Read the model definition and answer for the solid it produces. Units are mm, in the model's axes. Coordinates: 2 decimals unless noted, no trailing zeros. Write each loop counter-clockwise with the first axis right and the second up, starting at its lowest first coordinate (ties: lowest second). Pieces come first, ordered by that corner, then holes. Notation, with made-up numbers: M 83,74 L 114,74 A12 ccw 114,97 Z; hole C 69.5,-6 d8. An arc over 180 degrees is marked long. Write item = value, one per line.
from build123d import *

# Parameters (mm, degrees)
SKETCH1_R           = 4
BOSS_EXTRUDE1_DEPTH = 7
SKETCH2_R           = 3.375
CUT_EXTRUDE1_DEPTH  = 10
BOSS_EXTRUDE2_START = -0.25
SKETCH16_R          = 4.25
SKETCH16_R_2        = 4
BOSS_EXTRUDE2_DEPTH = 0.25


with BuildPart() as part:
    # Sketch1 → Boss-Extrude1 (new body)
    with BuildSketch(Plane(origin=(0, 0, 0), x_dir=(1, 0, 0), z_dir=(0, 1, 0))):
        with Locations(Location((0, 0, 0), (0, 0, 270))):
            Circle(SKETCH1_R)
    extrude(amount=BOSS_EXTRUDE1_DEPTH)

    # Sketch2 → Cut-Extrude1 (cut)
    with BuildSketch(Plane(origin=(0, 7, 0), x_dir=(1, 0, 0), z_dir=(0, 1, 0))):
        with Locations(Location((0, 0, 0), (0, 0, 270))):
            Circle(SKETCH2_R)
    extrude(amount=-CUT_EXTRUDE1_DEPTH, mode=Mode.SUBTRACT)

    # Sketch16 → Boss-Extrude2 (add)
    with BuildSketch(Plane(origin=(0, 7, 0), x_dir=(1, 0, 0), z_dir=(0, 1, 0)).offset(BOSS_EXTRUDE2_START)):
        with Locations(Location((0, 0, 0), (0, 0, 270))):
            Circle(SKETCH16_R)
        with Locations(Location((0, 0, 0), (0, 0, 270))):
            Circle(SKETCH16_R_2, mode=Mode.SUBTRACT)
    boss_extrude2 = extrude(amount=BOSS_EXTRUDE2_DEPTH)

    # Mirror1: Boss-Extrude2 across plane
    add(boss_extrude2.mirror(Plane.ZX.offset(3.5)))


solid = part.part
Item 1: Find section A-A (z = 0). Determine the outline of the cut face in (x, y) (3 decimals).
Worked answers:
outline = M -4.25,0 L -3.375,0 L -3.375,7 L -4.25,7 L -4.25,6.75 L -4,6.75 L -4,0.25 L -4.25,0.25 Z; M 3.375,0 L 4.25,0 L 4.25,0.25 L 4,0.25 L 4,6.75 L 4.25,6.75 L 4.25,7 L 3.375,7 Z
Item 2: Flat-ended cylindrical pins translate along their axes: pin 1 (2 mm diameter, centred on y = 4, z = -3, fed in from +X); pin 2 (3 mm diameter, centred on x = -2, y = 4, fed in from -Z); pin 3 (1 mm diameter, centred on x = 2, y = 5, fed in from +Z). Find the tip coordinate at first contact, or state that the pin passes through.
Worked answers:
pin_1 = 3.46
pin_2 = -3.97
pin_3 = 3.71
Item 3: Consider line 1 along X through (y, z) = (2, 0) (3 decimals); line 2 along Y through (x, z) = (3.25, 2.5); line 3 along Z through (x, y) = (-2, 2.25). Determine where each line is inside the solid, lowest interval first. Write a range as from..to.
Worked answers:
line_1 = -4..-3.375, 3.375..4
line_2 = 0..0.25, 6.75..7
line_3 = -3.46..-2.72, 2.72..3.46
Item 4: Find section C-C (y = 2.25). Determine the outline of the cut face in (x, z) (3 decimals), and give its area (3 significant figures).
Worked answers:
outline = C 0,0 d8; hole C 0,0 d6.75
area = 14.5 mm²
Item 5: For a pull along Y with two mould halves and no side action, classify faces 1 (the face through (2, 7, -3)), 2 (the face through (2, 0, -3)), 3 (the face through (-3.3, 3.5, -0.7)), 4 (the face through (-3.905, 3.454, -0.867)) as released by +Y, released by -Y, zero draft, split by the parting line, or undercut.
Worked answers:
face_1 = released by +Y
face_2 = released by -Y
face_3 = zero draft
face_4 = undercut
Item 6: Find section B-B (x = 0). Determine the outline of the cut face in (y, z) (3 decimals).
Worked answers:
outline = M 0,-4.25 L 0.25,-4.25 L 0.25,-4 L 6.75,-4 L 6.75,-4.25 L 7,-4.25 L 7,-3.375 L 0,-3.375 Z; M 0,3.375 L 7,3.375 L 7,4.25 L 6.75,4.25 L 6.75,4 L 0.25,4 L 0.25,4.25 L 0,4.25 Z
